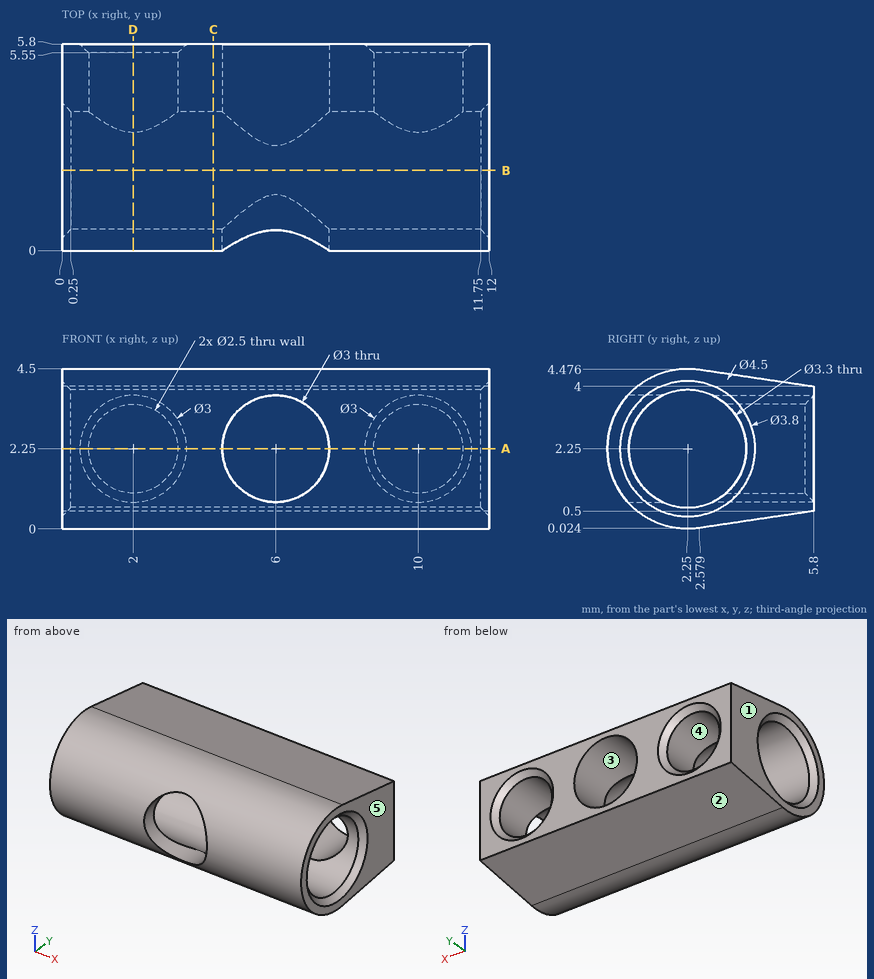
Verification items for this drawing (mm, ordinates from the low corner). A direction names the side the tool comes from. Give positions to 0.01 mm unless a question says otherwise; leave off trailing zeros. Loops run counter-clockwise (first coordinate to the right, second up) from the corner with the lowest first, then second, coordinate; pieces in that order, holes last. Notation, with made-up numbers: M -3.5,57.5 L 14.5,57.5 A17 cw 14.5,84.5 Z; hole C 68.5,31 d4. An arc over 180 degrees is marked long. Return JSON: item names as keys, results as strings. Group by question number.
1. Mould release check, pull along Z, two halves, no side actions. Record for the marked faces 1, 2 and 3: released by +Z, released by -Z, zero draft, split by the parting line, or undercut.
2. Thickness scan on L1, parallel to X at y = 4.65, z = 2.25; L2, parallel to X at y = 5.1, z = 1.65 (1 decimal); L3, parallel to Y at x = 8.5, z = 1.95. Record the ranges inside material, lowest first.
3. Tool access check on the marked faces 4 and 5. Record the directions out of +Z, -Z, +X, -X, +Y, -Y that give a thin tool (end or side, any length) a straight path to the whole face; none if there is none.
4. Cross-section at B-B on y = 2.25. Record the boundary of the cut face in (x, z), plus the area to 3 significant figures.
5. Cross-section at D-D on x = 2. Record the boundary of the cut face in (y, z).
6. Cross-section at A-A on z = 2.25. State how many separate pieces and enclosed holes the cut face has.
7. Cross-section at C-C on x = 4.25. Record the boundary of the cut face in (y, z).
8. Go/stop test with flat-tipped pins: pin 1 (1 mm diameter, centred on x = 8, y = 1.5, fed in from +Z); pin 2 (2 mm diameter, centred on x = 10, z = 2.25, fed in from +Y). Record where each tip stops, or that it passes through.
Return value:
{
 "1": {"face 1": "zero draft", "face 2": "released by -Z", "face 3": "undercut"},
 "2": {"L1": "0 to 0.75, 3.25 to 4.5, 7.5 to 8.75, 11.25 to 12", "L2": "0 to 0.9, 3.1 to 4.6, 7.4 to 8.9, 11.1 to 12", "L3": "0.02 to 0.63, 3.87 to 5.8"},
 "3": {"face 4": "+Y", "face 5": "+Z, -Z, +X, +Y, -Y"},
 "4": {"outline": "M 0,0 L 12,0 L 12,0.35 L 11.75,0.6 L 0.25,0.6 L 0,0.35 Z; M 0,4.15 L 0.25,3.9 L 11.75,3.9 L 12,4.15 L 12,4.5 L 0,4.5 Z", "area": "14.3 mm^2"},
 "5": {"outline": "M 2.58,0.02 L 5.8,0.5 L 5.8,0.75 L 5.55,1 L 3.33,1 A1.65 cw long 3.33,3.5 L 5.55,3.5 L 5.8,3.75 L 5.8,4 L 2.58,4.48 A2.25 ccw long Z"},
 "6": {"separate pieces": "6", "enclosed holes": "0"},
 "7": {"outline": "M 2.58,0.02 L 5.8,0.5 L 5.8,4 L 2.58,4.48 A2.25 ccw long Z; hole C 2.25,2.25 d3.3"},
 "8": {"pin 1": "z = 4.49", "pin 2": "y = 0.94"}
}
